Source: CAD feature listing. Evaluate the final solid. Frame: model axes, mm. Face numbers are marked on the shaded views. A direction names the side the tool comes from. Coordinates: 2 decimals unless noted, no trailing zeros. Order: outer loops, then holes, each group sorted by start corner. A loop starts at its lowest first (then second) coordinate and runs counter-clockwise, first axis right, second up. Notation, with made-up numbers: (-9, -40) - (11, -40) arc R29 ccw to (11, -14) - close; hole circle Ø8 at (-29.75, -31.5). An arc over 180 degrees is marked (long way). One line per question, with ' | ' between items.
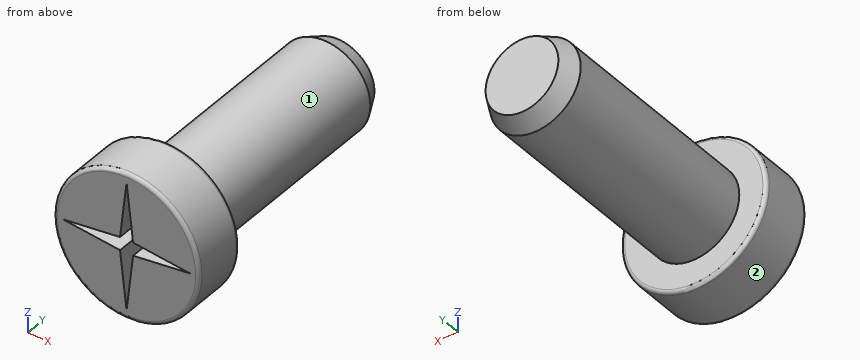
Autodesk Inventor part; units mm, degrees
ref_plane "YZ Plane" through (0, 0, 0) normal (1, 0, 0) x (0, 1, 0)
ref_plane "XZ Plane" through (0, 0, 0) normal (0, 1, 0) x (-1, 0, 0)
ref_plane "XY Plane" through (0, 0, 0) normal (0, 0, 1) x (1, 0, 0)
sketch "Sketch1" plane through (0, 0, 0) normal (0, 1, 0) x (-1, 0, 0)
  circle A0 centre (0, 0) radius 2.5
  circle A1 centre (0, 0) radius 4
  dimension "d0" = 5
  dimension "d1" = 8
extrude "Extrusion1" add sketch "Sketch1" along normal blind 15 contours A0
extrude "Extrusion2" add sketch "Sketch1" along normal blind 3
sketch "Sketch3" plane through (0, 0, 0) normal (0, -1, 0) x (1, 0, 0)
  line L0 (0, 0) -> (0, -0.4) construction
  circle A0 centre (0, 0) radius 4
  line L1 (4, 0) -> (3.5, 0) construction
  line L2 (0, 0) -> (0, 0.4) construction
  line L3 (0.359, 0.359) -> (3.5, 0)
  line L4 (3.5, 0) -> (0.359, -0.359)
  line L5 (0.359, -0.359) -> (0, -3.5)
  line L6 (-0.359, -0.359) -> (0, -3.5)
  line L7 (-0.359, -0.359) -> (-3.5, 0)
  line L8 (-3.5, 0) -> (-0.359, 0.359)
  line L9 (-0.359, 0.359) -> (0, 3.5)
  line L10 (0, 3.5) -> (0.359, 0.359)
  dimension "d14" = 0.4
  dimension "d15" = 0.5
  dimension "d16" = 0.4
  dimension "d21" = 103.04
  dimension "d22" = 103.04
  dimension "d23" = 13.04
  dimension "d24" = 3.1615
  dimension "d25" = 3.1615
extrude "Extrusion3" cut sketch "Sketch3" against normal blind 2 contours L3 L4 L5 L6 L7 L8 L9 L10
fillet "Fillet1" radius 0.2 2 edges at (4, 0, 0) (4, 3, 0)
thread "Thread1"
sketch "Sketch4" plane through (0, 15, 0) normal (0, 1, 0) x (1, 0, 0)
  circle A0 centre (0, 0) radius 2
  dimension "d31" = 4
extrude "Extrusion4" add sketch "Sketch4" along normal blind 1
loft "Loft1" add section 1 edges at (-2, 16, 0) section 2 edges at (2.5, 15, 0)
thread "Thread2"
properties part number "m5x12mmscrew"
(1) Pin query (flat end, axial travel): P1, Ø4, axis at x = -2, y = 5.5, coming from the +Z side. Return the tip coordinate at first contact, or that it passes through.
Taken from the geometry:
P1: stops at z = 2.5
(2) Cut plane B-B (y = 13). Return the cut outline in (x, z), and give its area (3 significant figures).
Taken from the geometry:
outline: circle Ø5 at (0, 0) | area: 19.6 mm²
(3) Material intervals for L1, parallel to Y at x = -1.5, z = 2.25; L2, parallel to Z at x = 1.5, y = 7.75; L3, parallel to X at y = 7.75, z = 0, sorted ascending. Write a range as from..to.
Taken from the geometry:
L1: y = 0..3 | L2: z = -2..2 | L3: x = -2.5..2.5
(4) Cut plane A-A (y = 2.5). Return the cut outline in (x, z), and give its area (3 significant figures).
Taken from the geometry:
outline: circle Ø8 at (0, 0) | area: 50.3 mm²
(5) Set-up query: the marked faces 1 and 2. Return all of +Z, -Z, +X, -X, +Y, -Y with unobstructed straight access to the full face (end or side cutting, diameter ignored); none if empty.
Taken from the geometry:
face 1: +Y | face 2: +Y, -Y
